Verification items for the finished model (mm, model axes). Round coordinates to 2 decimals unless told otherwise and drop trailing zeros. Order: outer loops, then holes, each group sorted by start corner. A loop starts at its lowest first (then second) coordinate and runs counter-clockwise, first axis right, second up. Notation, with made-up numbers: (63, 40) -> (110, 40) arc R29 ccw to (110, 77) -> close; hole circle Ø10 at (56, 7). An arc over 180 degrees is marked (long way). Return JSON: item names as keys, results as strings. Group by question number.
Item 1: Draft check along Y on faces 1 (the flat face through (-2, 2, 0)), 2 (the flat face through (0, 0, 7)), 3 (the flat face through (0, 0, 8.5)), 4 (the cylindrical face through (9.54, 3, 8.2)). Enter one of: pulls with the +Y half, pulls with the -Y half, needs draft (parallel to the pull), parting line crosses it, or undercut.
Item 2: Depth check by flat-ended pin: pin 1 Ø3 at (x, y) = (7.5, -2.5) entering from -Z; pin 2 Ø4 at (x, z) = (-3, 2.5) entering from +Y. Enter the tip coordinate at first touch or a pass-through.
Item 3: Sectioned sample at A-A on z = 6.5. Record the cut outline in (x, y).
Item 4: Scan lines: probe 1 along Y at (x, z) = (0, 5.5); probe 2 along Z at (x, y) = (6.75, -3); probe 3 along X at (y, z) = (1.5, 6.25). Record each from-to range of solid material in increasing order. Write a range as from..to.
```python
from build123d import *

# Parameters (mm, degrees)
CYLINDER_R     = 2.5
CYLINDER_DEPTH = 7
FILLET_1_R     = 5
FILLET_2_R     = 0.5


with BuildPart() as pocket:
    # Cylinder → Cylinder (new body)
    with BuildSketch(Plane.XY):
        Circle(CYLINDER_R)
    extrude(amount=CYLINDER_DEPTH)


with BuildPart() as handle:
    # Sketch → Revolution (revolve)
    with BuildSketch(Plane.XZ):
        with BuildLine():
            Line((0, 0), (4, 0))
            Line((4, 0), (4, 7))
            Line((4, 7), (8, 7))
            Line((8, 7), (10, 7.5))
            Line((10, 7.5), (10, 8.499999))
            ThreePointArc((10, 8.499999), (9.500011, 9), (9, 8.500022))
            Line((9, 8.5), (9, 8.500022))
            Line((0, 8.5), (9, 8.5))
            Line((0, 8.5), (0, 0))
        make_face()
    revolve(axis=Axis((0, 0, 0), (0, 0, 1)))

    # Fillet 1
    fillet_1_edges = [handle.edges().sort_by_distance(p)[0] for p in [
        (-8, 0, 7),
    ]]
    fillet(fillet_1_edges, radius=FILLET_1_R)

    # Fillet 2
    fillet_2_edges = [handle.edges().sort_by_distance(p)[0] for p in [
        (-10, 0, 7.5),
    ]]
    fillet(fillet_2_edges, radius=FILLET_2_R)

    # Cut: cut Pocket
    add(pocket.part, mode=Mode.SUBTRACT)


solid = handle.part
```
Recorded:
{
 "1": {"face 1": "needs draft", "face 2": "undercut", "face 3": "undercut", "face 4": "parting line crosses it"},
 "2": {"pin 1": "z = 7", "pin 2": "y = 3.87"},
 "3": {"outline": "circle Ø8 at (0, 0); hole circle Ø5 at (0, 0)"},
 "4": {"probe 1": "-4..-2.5, 2.5..4", "probe 2": "7..8.5", "probe 3": "-3.71..-2, 2..3.71"}
}
